from build123d import *

# Parameters (mm, degrees)
CROQUIS1_W              = 150
CROQUIS1_H              = 10
CROQUIS1_R              = 2.5
SALIENTE_EXTRUIR1_DEPTH = 4
REDONDEO1_R             = 4


with BuildPart() as part:
    # Croquis1 → Saliente-Extruir1 (new body)
    with BuildSketch(Plane(origin=(0, 0, 0), x_dir=(1, 0, 0), z_dir=(0, 1, 0))):
        Rectangle(CROQUIS1_W, CROQUIS1_H)
        with Locations((-70, 0)):
            Circle(CROQUIS1_R, mode=Mode.SUBTRACT)
        with Locations((70, 0)):
            Circle(CROQUIS1_R, mode=Mode.SUBTRACT)
        Circle(CROQUIS1_R, mode=Mode.SUBTRACT)
    extrude(amount=SALIENTE_EXTRUIR1_DEPTH)

    # Redondeo1
    redondeo1_edges = [part.edges().sort_by_distance(p)[0] for p in [
        (75, 2, 5),
        (-75, 2, 5),
        (-75, 2, -5),
        (75, 2, -5),
    ]]
    fillet(redondeo1_edges, radius=REDONDEO1_R)


solid = part.part
Part model, mm, in its own coordinate system. Coordinates: 2 decimals unless noted, no trailing zeros. Loops run counter-clockwise (first coordinate to the right, second up) from the corner with the lowest first, then second, coordinate; pieces in that order, holes last. Notation, with made-up numbers: (-13.5, -13.75) -> (40.5, -13.75) arc R7 cw to (40.5, -4.75) -> close; hole circle Ø9 at (-24.5, 26). An arc over 180 degrees is marked (long way). Use a Markdown table: item, result. Add a question column.
Item 1: Probe probe 1 along X at (y, z) = (1.1, 0); probe 2 along Z at (x, y) = (70, 1.25); probe 3 along X at (y, z) = (1, 2.25). List the from-to ranges inside material, lowest first.
Item 2: Flat gauge pin, fed straight in: P1, Ø4, axis at x = -70, z = 0, coming from the -Y side. Where does the tip first touch, or does it go through?
Item 3: Band-saw the part on B-B on x = 0. Write the cut outline in (y, z).
Item 4: Pull direction Z, two halves, no side cores. Call faces 1 (the flat face through (-1, 4, -3)), 2 (the cylindrical face through (-73.859, 2.028, 3.797)), 3 (the cylindrical face through (-73.859, 2.028, -3.797)), 4 (the cylindrical face through (-72, 2, 1.5)): +Z half, -Z half, draft (parallel to the pull), parting line (faces both ways), or undercut.
Item 5: Band-saw the part on A-A on y = 2.1. Write the cut outline in (x, z), plus the area to 3 significant figures.
Geometry says:
| question | item | result |
|---|---|---|
| 1 | probe 1 | -75 to -72.5, -67.5 to -2.5, 2.5 to 67.5, 72.5 to 75 |
| 1 | probe 2 | -5 to -2.5, 2.5 to 5 |
| 1 | probe 3 | -74.8 to -71.09, -68.91 to -1.09, 1.09 to 68.91, 71.09 to 74.8 |
| 2 | P1 | through |
| 3 | outline | (0, -5) -> (4, -5) -> (4, -2.5) -> (0, -2.5) -> close; (0, 2.5) -> (4, 2.5) -> (4, 5) -> (0, 5) -> close |
| 4 | face 1 | draft |
| 4 | face 2 | +Z half |
| 4 | face 3 | -Z half |
| 4 | face 4 | undercut |
| 5 | outline | (-75, -1) arc R4 ccw to (-71, -5) -> (71, -5) arc R4 ccw to (75, -1) -> (75, 1) arc R4 ccw to (71, 5) -> (-71, 5) arc R4 ccw to (-75, 1) -> close; hole circle Ø5 at (-70, 0); hole circle Ø5 at (0, 0); hole circle Ø5 at (70, 0) |
| 5 | area | 1,430 mm² |
